Source: three-view drawing plus pictorial views. Frame: mm from the lowest corner of the part. A direction names the side the tool comes from. Give positions to 0.01 mm unless a question says otherwise; leave off trailing zeros. Loops run counter-clockwise (first coordinate to the right, second up) from the corner with the lowest first, then second, coordinate; pieces in that order, holes last.
1. Section D-D, the plane x = 3.65. Output: boundary loops of the cut face in (y, z), then the cut area to 3 significant figures.
2. Section C-C, the plane y = 3.45. Output: boundary loops of the cut face in (x, z).
3. First-contact query: P1, Ø1, axis at x = 3, z = 2, coming from the -Y side; P2, Ø2, axis at y = 2.5, z = 4, coming from the -X side; P3, Ø1, axis at x = 2.5, y = 1.5, coming from the +Z side. Flat tips, straight axial feed; report the tip coordinate or a pass-through.
4. Access query for the marked faces 1 and 2. Directions: +Z, -Z, +X, -X, +Y, -Y. A direction counts if a zero-diameter tool reaches every point of the face in a straight line with its end or side. Return the directions, or none.
5. Section A-A, the plane z = 2.4. Output: boundary loops of the cut face in (x, y).
6. Draft query along X for the marked faces 3, 4 and 5. Return one class per face: +X half, -X half, draft (parallel to the pull), parting line (faces both ways), or undercut.
7. Section B-B, the plane z = 1.2. Output: boundary loops of the cut face in (x, y).
8. Material intervals for line 1 along Z through (x, y) = (0.7, 2); line 2 along X through (y, z) = (1.1, 3.95); line 3 along Z through (x, y) = (3.8, 2.6), sorted ascending.
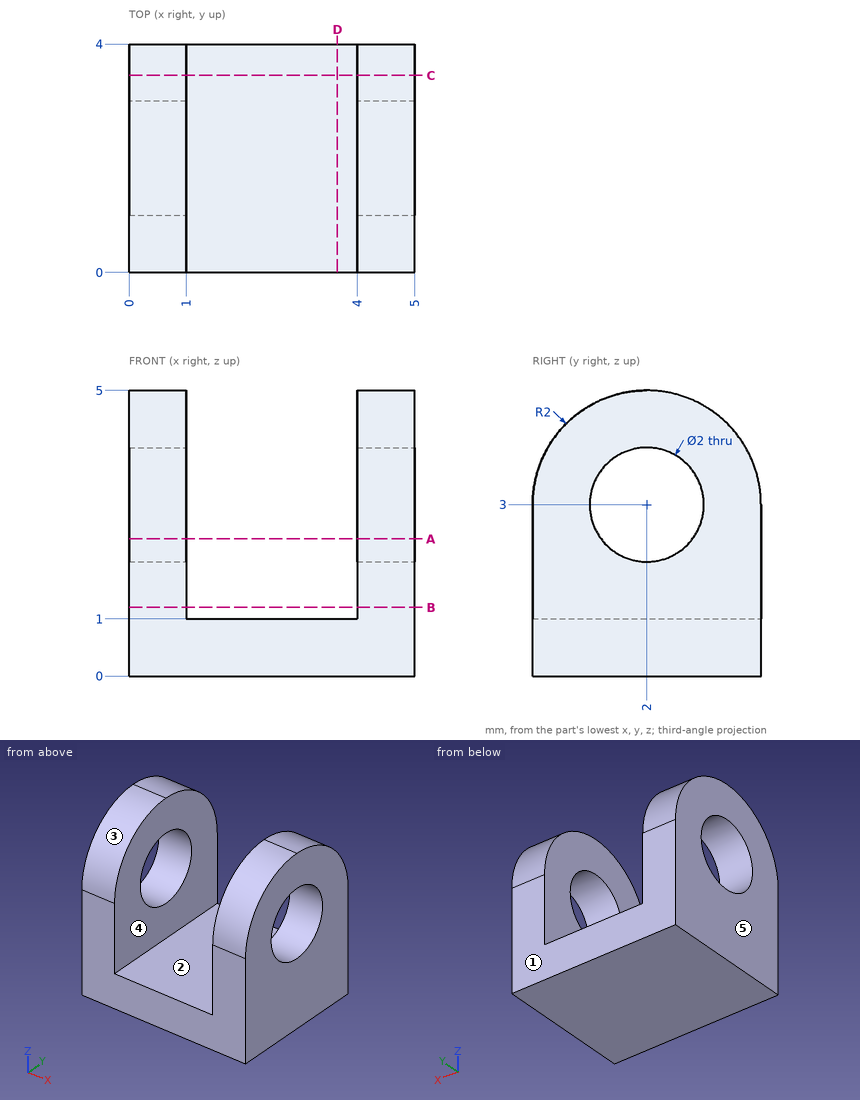
Answers below:
1. outline: (0, 0) - (4, 0) - (4, 1) - (0, 1) - close
1. area: 4.00 mm2
2. outline: (0, 0) - (5, 0) - (5, 4.38) - (4, 4.38) - (4, 1) - (1, 1) - (1, 4.38) - (0, 4.38) - close
3. P1: passes through
3. P2: stops at x = 0
3. P3: stops at z = 1
4. face 1: +Z, -Z, +X, -X, +Y
4. face 2: +Z, +Y, -Y
5. outline: (0, 0) - (1, 0) - (1, 1.2) - (0, 1.2) - close; (0, 2.8) - (1, 2.8) - (1, 4) - (0, 4) - close; (4, 0) - (5, 0) - (5, 1.2) - (4, 1.2) - close; (4, 2.8) - (5, 2.8) - (5, 4) - (4, 4) - close
6. face 3: draft
6. face 4: undercut
6. face 5: -X half
7. outline: (0, 0) - (1, 0) - (1, 4) - (0, 4) - close; (4, 0) - (5, 0) - (5, 4) - (4, 4) - close
8. line 1: z = 0 to 2, 4 to 5
8. line 2: x = 0 to 1, 4 to 5
8. line 3: z = 0 to 1
